Autodesk Inventor part; units mm, degrees
ref_plane "Endfläche-ProbeHeadarme" through (0, 0, -86) normal (0, 0, 1) x (1, 0, 0)
ref_plane "Z-LowerBelt" through (0, 0, -49.1) normal (0, 0, 1) x (1, 0, 0)
ref_plane "X-Belts" through (26.75, 0, 0) normal (1, 0, 0) x (0, 1, 0)
sketch "S-ProbeHead-BaseSkizze" plane through (0, 0, 0) normal (0, 0, 1) x (1, 0, 0)
  line L0 (-40, 40) -> (40, 40)
  line L1 (40, 40) -> (40, -40)
  line L2 (40, -40) -> (-40, -40)
  line L3 (-40, -40) -> (-40, 40)
  line L4 (-40, 40) -> (40, -40) construction
  line L5 (40, 40) -> (-40, -40) construction
  line L6 (-56.34, 0) -> (58.04, 0) construction
  circle A0 centre (-30, 0) radius 5
  line L7 (0, 83.0683) -> (0, -88.0384) construction
  line L8 (-7.5, 58.6245) -> (-7.5, -60.8735) construction
  line L9 (-16, 21) -> (16, 21) construction
  line L10 (16, 21) -> (16, -21) construction
  line L11 (16, -21) -> (-16, -21) construction
  line L12 (-16, -21) -> (-16, 21) construction
  line L13 (-16, 21) -> (16, -21) construction
  line L14 (16, 21) -> (-16, -21) construction
  circle A1 centre (-12.5, -10) radius 1.65
  circle A2 centre (-12.5, 10) radius 1.65
  circle A3 centre (12.5, -10) radius 1.65
  circle A4 centre (12.5, 10) radius 1.65
  line L15 (-20, 57.6709) -> (-20, -63.5946)
  line L16 (7.5, 58.6245) -> (7.5, -60.8735) construction
  line L17 (20, 57.6709) -> (20, -63.5946)
  line L18 (41.7, 25) -> (-40, 25)
  line L19 (-40, 25) -> (-40, -25)
  line L20 (-40, -25) -> (41.7, -25)
  line L21 (41.7, -25) -> (41.7, 25)
  line L22 (22, 25) -> (22, -25)
  line L23 (-22, -25) -> (-22, 25)
  point P0 (0, 0)
  point P1 (41.7, 0)
  dimension "d1" = 80
  dimension "d2" = 80
  dimension "d4" = 10
  dimension "d6" = 30
  dimension "d20" = 7.5
  dimension "d21" = 32
  dimension "d22" = 42
  dimension "d23" = 3.3
  dimension "d24" = 10
  dimension "d25" = 12.5
  dimension "d26" = 20
  dimension "d27" = 50
  dimension "d30" = 20
  dimension "d31" = 21.7
  dimension "d32" = 2
  dimension "d37" = 2
extrude "BasePlate" add sketch "S-ProbeHead-BaseSkizze" along normal blind 4 contours L18 L23 L20 L3 | L18 L17 L20 L15 | L15 L20 L23 L18 | L18 L22 L20 L17 | L18 L21 L20 L1 | L1 L20 L22 L18
ref_plane "Endfläche-ProbeHeadarme" through (0, 0, -86) normal (0, 0, 1) x (1, 0, 0)
ref_plane "ProfilDownside" through (0, 0, -56) normal (0, 0, 1) x (1, 0, 0)
extrude "Arms" add sketch "S-ProbeHead-BaseSkizze" against normal up to surface (86 mm away) contours L18 L23 L20 L3 | L18 L21 L20 L1 | L1 L20 L22 L18
ref_plane "Z-UpperBelt" through (0, 0, -36.1) normal (0, 0, 1) x (1, 0, 0)
ref_plane "Z-LowerBelt" through (0, 0, -49.1) normal (0, 0, 1) x (1, 0, 0)
ref_plane "X-Belts" through (26.75, 0, 0) normal (1, 0, 0) x (0, 1, 0)
sketch "S-Tensioners" plane through (-40, -25, 4) normal (0, -1, 0) x (1, 0, 0)
  line L0 (64.75, -47.5) -> (78.95, -47.5)
  line L1 (78.95, -47.5) -> (78.95, -58.7)
  line L2 (78.95, -58.7) -> (64.75, -58.7)
  line L3 (64.75, -58.7) -> (64.75, -47.5)
  line L4 (64.75, -47.5) -> (78.95, -58.7) construction
  line L5 (78.95, -47.5) -> (64.75, -58.7) construction
  line L6 (71.85, -74) -> (71.85, 12.5724) construction
  line L7 (-16.34, -40.1) -> (98.04, -40.1) construction
  line L8 (-16.34, -53.1) -> (98.04, -53.1) construction
  circle A0 centre (74.15, -53.1) radius 2.65
  line L9 (64.75, -34.5) -> (78.95, -34.5)
  line L10 (78.95, -34.5) -> (78.95, -45.7)
  line L11 (78.95, -45.7) -> (64.75, -45.7)
  line L12 (64.75, -45.7) -> (64.75, -34.5)
  line L13 (64.75, -34.5) -> (78.95, -45.7) construction
  line L14 (78.95, -34.5) -> (64.75, -45.7) construction
  circle A1 centre (74.15, -40.1) radius 2.65
  circle A2 centre (74.15, -40.1) radius 4.5
  circle A3 centre (74.15, -53.1) radius 4.5
  line L15 (66.75, 33.0869) -> (66.75, -110.5145) construction
  point P0 (40, -4)
  point P1 (78.95, -40.1)
  point P2 (78.95, -53.1)
  dimension "d38" = 14.2
  dimension "d39" = 11.2
  dimension "d42" = 5.3
  dimension "d43" = 14.2
  dimension "d44" = 11.2
  dimension "d45" = 5.3
  dimension "d53" = 4.8
  dimension "d54" = 4.8
  dimension "d55" = 9
  dimension "d56" = 9
  dimension "d58" = 7.4
  dimension "d59" = 7.4
extrude "Ex-Tensioners1-Holes" cut sketch "S-Tensioners" against normal blind 50 contours A0 | A1
extrude "Ex-Tensioners2-SlideVolume" cut sketch "S-Tensioners" along normal blind 35 from surface at -50 contours L0 L1 L2 L3 | A3
extrude "Ex-Tensioners3-SlideVolume" cut sketch "S-Tensioners" against normal blind 35 contours L9 L10 L11 L12 | A2
extrude "Ex-Tensioners4-SrewHead" cut sketch "S-Tensioners" against normal blind 7 contours A3
extrude "Ex-Tensioners5-SrewHead" cut sketch "S-Tensioners" along normal blind 7 from surface at -50 contours A2
sketch "S-Anschraubpunkte-ProbeAntenna" plane through (0, 0, -86) normal (0, 0, 1) x (1, 0, 0)
  line L0 (-56.34, 0) -> (58.04, 0) construction
  line L1 (0, 35) -> (0, -35) construction
  line L2 (41.7, 25) -> (-40, 25)
  line L3 (41.7, -25) -> (41.7, 25)
  line L4 (-40, -25) -> (41.7, -25)
  line L5 (-40, 25) -> (-40, -25)
  line L6 (41.7, 25) -> (26.7, 25)
  line L7 (26.7, 25) -> (26.7, 40)
  line L8 (26.7, 40) -> (41.7, 40)
  line L9 (41.7, 40) -> (41.7, 25)
  line L10 (22, -25) -> (22, 25)
  line L11 (22, 25) -> (22, -25)
  line L12 (-22, 25) -> (-22, -25)
  line L13 (-22, -25) -> (-22, 25)
  line L14 (41.7, 32.5) -> (26.7, 32.5) construction
  line L15 (34.2, 40) -> (34.2, 25) construction
  circle A0 centre (34.2, 32.5) radius 2.15
  circle A1 centre (34.2, 32.5) radius 4
  line L16 (0.85, 53.9557) -> (0.85, -47.9335) construction
  line L17 (-40, 25) -> (-25, 25)
  line L18 (-25, 25) -> (-25, 40)
  line L19 (-25, 40) -> (-40, 40)
  line L20 (-40, 40) -> (-40, 25)
  circle A2 centre (-32.5, 32.5) radius 2.15
  circle A3 centre (-32.5, 32.5) radius 4
  line L21 (41.7, -25) -> (26.7, -25)
  line L22 (26.7, -25) -> (26.7, -40)
  line L23 (26.7, -40) -> (41.7, -40)
  line L24 (41.7, -40) -> (41.7, -25)
  circle A4 centre (34.2, -32.5) radius 2.15
  circle A5 centre (34.2, -32.5) radius 4
  line L25 (-40, -40) -> (-40, -25)
  line L26 (-25, -40) -> (-40, -40)
  line L27 (-40, -25) -> (-25, -25)
  line L28 (-25, -25) -> (-25, -40)
  circle A6 centre (-32.5, -32.5) radius 4
  circle A7 centre (-32.5, -32.5) radius 2.15
  point P0 (0, 0)
  dimension "d67" = 15
  dimension "d68" = 15
  dimension "d69" = 4.3
  dimension "d70" = 8
  dimension "d71" = 81.7
  dimension "d72" = 40.85
  dimension "d75" = 65
  dimension "d76" = 66.7
extrude "Ex-Anschraubpunkte-M4" add sketch "S-Anschraubpunkte-ProbeAntenna" along normal blind 7 contours L2 L7 L8 L9 | L24 L23 L22 L4 | L2 L20 L19 L18 | L28 L26 L25 L4 | A1 | A3 | A5 | A6
extrude "Ex-Anschraubpunkt-M4-ScrewHead" cut sketch "S-Anschraubpunkte-ProbeAntenna" against normal blind 3 from surface at 7 contours A1 | A3 | A5 | A6
ref_plane "ProfilTopSide" through (0, 0, -16) normal (0, 0, 1) x (1, 0, 0)
equation "\"d43\" = d38"
equation "\"d44\" = d39"
equation "\"d45\" = d42"
equation "\"d53\" = d54"
equation "\"d55\" = d56"
equation "\"d58\" = d59"
equation "\"d72\" = 0.5 * d71"
properties part number "ProbeHead-BaseBody V1"
The model under review builds one solid part; all positions refer to its coordinate system, in mm. A direction names the side the tool comes from. Give positions to 0.01 mm unless a question says otherwise; leave off trailing zeros. Loops run counter-clockwise (first coordinate to the right, second up) from the corner with the lowest first, then second, coordinate; pieces in that order, holes last. Notation, with made-up numbers: (61.25, 17.25) -> (116.25, 17.25) arc R29 cw to (116.25, 55.25) -> close; hole circle Ø1 at (48, 67.5). An arc over 180 degrees is marked (long way). Answer as a JSON object with one key per item and string values. Group by question number.
Q1. Take a section at B-B (x = 12.5). Write out the cut boundary in (y, z), plus the area to 3 significant figures.
Q2. Tool access review of faces 1 (the flat face through (22, 0, -42)), 2 (the flat face through (37, 36, -79)), 3 (the cylindrical face through (36.35, -29.127, -80.479)), 4 (the flat face through (-25, -32, -83)): name each direction out of +Z, -Z, +X, -X, +Y, -Y from which nothing blocks a thin tool from reaching the whole face with its end or side.
Q3. Take a section at D-D (z = -36.1). Write out the cut boundary in (x, y).
Q4. Draft analysis for pull direction Y (two halves, no side actions). For faces 5 (the flat face through (24.75, -8, -36)), 6 (the cylindrical face through (-33.021, -28.534, -80.479)), 7 (the flat face through (34, -18, -52)), state which applies: pulls with the +Y half, pulls with the -Y half, needs draft (parallel to the pull), parting line crosses it, or undercut.
Q5. Take a section at A-A (y = -32.5). Write out the cut boundary in (x, z).
Q6. Insertion check: pin 1 (5.5 mm diameter, centred on x = -32.5, y = 32.5, fed in from +Z); pin 2 (12 mm diameter, centred on x = 25, z = -63.5, fed in from -Y); pin 3 (3.5 mm diameter, centred on x = 34.5, z = -34.5, fed in from -Y); pin 4 (7 mm diameter, centred on x = -32.5, y = -32.5, fed in from -Z). Each pin has a flat end and moves straight along its axis. Give the tip position at first contact, or say it passes through.
Q7. Take a section at C-C (z = -7). Write out the cut boundary in (x, y), plus the area to 3 significant figures.
Q8. Wall thickness on line 1 along X through (y, z) = (9, -34); line 2 along Z through (x, y) = (34, -12); line 3 along X through (y, z) = (24, -12): over which ranges is each line inside the solid? List them lowest first.
Answer below:
{
 "1": {"outline": "(-25, 0) -> (-11.65, 0) -> (-11.65, 4) -> (-25, 4) -> close; (-8.35, 0) -> (8.35, 0) -> (8.35, 4) -> (-8.35, 4) -> close; (11.65, 0) -> (25, 0) -> (25, 4) -> (11.65, 4) -> close", "area": "174 mm2"},
 "2": {"face 1": "-Z, +Y, -Y", "face 2": "+Z, +X, -X, +Y", "face 3": "+Z", "face 4": "+Z, -Z, -Y"},
 "3": {"outline": "(-40, -25) -> (-22, -25) -> (-22, 25) -> (-40, 25) -> close; (22, -25) -> (24.75, -25) -> (24.75, 10) -> (31.5, 10) -> (31.5, 18) -> (29.65, 18) -> (29.65, 25) -> (22, 25) -> close; (36.8, 10) -> (38.95, 10) -> (38.95, -25) -> (41.7, -25) -> (41.7, 25) -> (38.65, 25) -> (38.65, 18) -> (36.8, 18) -> close; hole circle Ø10 at (-30, 0)"},
 "4": {"face 5": "needs draft", "face 6": "undercut", "face 7": "pulls with the -Y half"},
 "5": {"outline": "(-40, -86) -> (-34.65, -86) -> (-34.65, -82) -> (-36.5, -82) -> (-36.5, -79) -> (-40, -79) -> close; (-30.35, -86) -> (-25, -86) -> (-25, -79) -> (-28.5, -79) -> (-28.5, -82) -> (-30.35, -82) -> close; (26.7, -86) -> (32.05, -86) -> (32.05, -82) -> (30.2, -82) -> (30.2, -79) -> (26.7, -79) -> close; (36.35, -86) -> (41.7, -86) -> (41.7, -79) -> (38.2, -79) -> (38.2, -82) -> (36.35, -82) -> close"},
 "6": {"pin 1": "stops at z = -82", "pin 2": "stops at y = -25", "pin 3": "stops at y = 10", "pin 4": "stops at z = -86"},
 "7": {"outline": "(-40, -25) -> (-22, -25) -> (-22, 25) -> (-40, 25) -> close; (22, -25) -> (41.7, -25) -> (41.7, 25) -> (22, 25) -> close; hole circle Ø10 at (-30, 0)", "area": "1,810 mm2"},
 "8": {"line 1": "x = -40 to -22, 22 to 24.75, 38.95 to 41.7", "line 2": "z = -86 to -51.75, -46.45 to -41.7, -30.5 to 4", "line 3": "x = -40 to -22, 22 to 41.7"}
}
